Can you work these out from the model? Positions are in its coordinate system, mm. Round coordinates to 2 decimals unless told otherwise and drop trailing zeros. Order: outer loops, then holes, each group sorted by start corner. A loop starts at its lowest first (then second) coordinate and runs counter-clockwise, first axis right, second up. Notation, with made-up numbers: (7, 78.5) -> (38, 78.5) arc R18 ccw to (38, 106.5) -> close; hole circle Ø10 at (62.25, 43). An arc over 180 degrees is marked (long way). Use a Markdown table: item, result. Add a question column.
Q1. If we section it at B-B on y = 19.5: List the corners of the cut face in (x, z) for me.
Q2. I need wall thicknesses on line 1 along Y through (x, z) = (-55, 0.6); line 2 along Y through (x, z) = (33, 0.7) (3 decimals); line 3 along Y through (x, z) = (131.5, 0.3). Which ranges of each line are inside material? Lowest first, please. Write a range as [from, to].
Q3. If we section it at C-C on z = 0.4: Give the number of separate pieces and of enclosed holes in the cut face, plus the area to 3 significant figures.
Q4. If we section it at A-A on x = 22: List the corners of the cut face in (y, z) for me.
Q5. We'd pull the mould along Y, two halves only. Please class faces 1 (the face through (132.801, 134.024, 0.986)), 2 (the face through (2, 162, 0)): +Y half, -Y half, draft (parallel to the pull), parting line (faces both ways), or undercut.
```python
from build123d import *

# Parameters (mm, degrees)
SKETCH_1_R      = 2.05
SKETCH_1_R_2    = 4
SKETCH_1_W      = 8.8
SKETCH_1_H      = 2.8
SKETCH_1_W_2    = 2.5
SKETCH_1_H_2    = 8.5
SKETCH_1_W_3    = 8.5
SKETCH_1_H_3    = 2.5
SKETCH_1_W_4    = 241.301375666
SKETCH_1_H_4    = 241.301375666
SKETCH_1_H_5    = 67.3
EXTRUDE_1_DEPTH = 2


with BuildPart() as part:
    # 草图1 → 凸台-拉伸1 (new body)
    with BuildSketch(Plane.XY):
        Polygon((150.650687833, -150.650687833), (-150.650687833, -150.650687833), (-150.650687833, 150.650687833), (-150.650687833, 277.950687833), (150.650687833, 277.950687833), (150.650687833, 150.650687833), align=None)
        with Locations((0.724285714, -142.895)):
            Circle(SKETCH_1_R, mode=Mode.SUBTRACT)
        with Locations((66.724285714, -142.895)):
            Circle(SKETCH_1_R, mode=Mode.SUBTRACT)
        with Locations(Location((-65.275714286, -142.895, 0), (0, 0, 180))):
            Circle(SKETCH_1_R, mode=Mode.SUBTRACT)
        with Locations(Location((-143.125714286, 66.955, 0), (0, 0, 180))):
            Circle(SKETCH_1_R, mode=Mode.SUBTRACT)
        with Locations((-143.125714286, 0.955)):
            Circle(SKETCH_1_R, mode=Mode.SUBTRACT)
        with Locations((-143.125714286, -65.045)):
            Circle(SKETCH_1_R, mode=Mode.SUBTRACT)
        with Locations(Location((66.874285714, 144.955, 0), (0, 0, 180))):
            Circle(SKETCH_1_R, mode=Mode.SUBTRACT)
        with Locations((0.874285714, 144.955)):
            Circle(SKETCH_1_R, mode=Mode.SUBTRACT)
        with Locations((-65.125714286, 144.955)):
            Circle(SKETCH_1_R, mode=Mode.SUBTRACT)
        with Locations(Location((144.874285714, -65.045, 0), (0, 0, 180))):
            Circle(SKETCH_1_R, mode=Mode.SUBTRACT)
        with Locations((144.874285714, 0.955)):
            Circle(SKETCH_1_R, mode=Mode.SUBTRACT)
        with Locations((144.874285714, 66.955)):
            Circle(SKETCH_1_R, mode=Mode.SUBTRACT)
        with Locations((-130.650687833, -130.650687833)):
            Circle(SKETCH_1_R_2, mode=Mode.SUBTRACT)
        with Locations((-130.650687833, 130.650687833)):
            Circle(SKETCH_1_R_2, mode=Mode.SUBTRACT)
        with Locations((130.650687833, 130.650687833)):
            Circle(SKETCH_1_R_2, mode=Mode.SUBTRACT)
        with Locations((130.650687833, -130.650687833)):
            Circle(SKETCH_1_R_2, mode=Mode.SUBTRACT)
        with Locations((99.724285714, -142.895)):
            Rectangle(SKETCH_1_W, SKETCH_1_H, mode=Mode.SUBTRACT)
        with Locations((33.724285714, -142.895)):
            Rectangle(SKETCH_1_W, SKETCH_1_H, mode=Mode.SUBTRACT)
        with Locations((-32.275714286, -142.895)):
            Rectangle(SKETCH_1_W, SKETCH_1_H, mode=Mode.SUBTRACT)
        with Locations((-98.275714286, -142.895)):
            Rectangle(SKETCH_1_W, SKETCH_1_H, mode=Mode.SUBTRACT)
        with Locations((-143.125714286, 99.955)):
            Rectangle(SKETCH_1_W_2, SKETCH_1_H_2, mode=Mode.SUBTRACT)
        with Locations((-143.125714286, 33.955)):
            Rectangle(SKETCH_1_W_2, SKETCH_1_H_2, mode=Mode.SUBTRACT)
        with Locations((-143.125714286, -32.045)):
            Rectangle(SKETCH_1_W_2, SKETCH_1_H_2, mode=Mode.SUBTRACT)
        with Locations((-143.125714286, -98.045)):
            Rectangle(SKETCH_1_W_2, SKETCH_1_H_2, mode=Mode.SUBTRACT)
        with Locations((99.874285714, 144.955)):
            Rectangle(SKETCH_1_W_3, SKETCH_1_H_3, mode=Mode.SUBTRACT)
        with Locations((33.874285714, 144.955)):
            Rectangle(SKETCH_1_W_3, SKETCH_1_H_3, mode=Mode.SUBTRACT)
        with Locations((-32.125714286, 144.955)):
            Rectangle(SKETCH_1_W_3, SKETCH_1_H_3, mode=Mode.SUBTRACT)
        with Locations((-98.125714286, 144.955)):
            Rectangle(SKETCH_1_W_3, SKETCH_1_H_3, mode=Mode.SUBTRACT)
        with Locations((144.874285714, -98.045)):
            Rectangle(SKETCH_1_W_2, SKETCH_1_H_2, mode=Mode.SUBTRACT)
        with Locations((144.874285714, -32.045)):
            Rectangle(SKETCH_1_W_2, SKETCH_1_H_2, mode=Mode.SUBTRACT)
        with Locations((144.874285714, 33.955)):
            Rectangle(SKETCH_1_W_2, SKETCH_1_H_2, mode=Mode.SUBTRACT)
        with Locations((144.874285714, 99.955)):
            Rectangle(SKETCH_1_W_2, SKETCH_1_H_2, mode=Mode.SUBTRACT)
        Rectangle(SKETCH_1_W_4, SKETCH_1_H_4, mode=Mode.SUBTRACT)
        with Locations((0, 214.300687833)):
            Rectangle(SKETCH_1_W_4, SKETCH_1_H_5, mode=Mode.SUBTRACT)
    extrude(amount=EXTRUDE_1_DEPTH)


solid = part.part
```
Answer below:
| question | item | result |
|---|---|---|
| 1 | outline | (-150.65, 0) -> (-120.65, 0) -> (-120.65, 2) -> (-150.65, 2) -> close; (120.65, 0) -> (150.65, 0) -> (150.65, 2) -> (120.65, 2) -> close |
| 2 | line 1 | [-150.65, -120.65], [120.65, 180.65], [247.95, 277.95] |
| 2 | line 2 | [-150.651, -144.295], [-141.495, -120.651], [120.651, 143.705], [146.205, 180.651], [247.951, 277.951] |
| 2 | line 3 | [-150.65, -134.56], [-126.74, 126.74], [134.56, 277.95] |
| 3 | separate pieces | 1 |
| 3 | enclosed holes | 34 |
| 3 | area | 54,000 mm² |
| 4 | outline | (-150.65, 0) -> (-120.65, 0) -> (-120.65, 2) -> (-150.65, 2) -> close; (120.65, 0) -> (180.65, 0) -> (180.65, 2) -> (120.65, 2) -> close; (247.95, 0) -> (277.95, 0) -> (277.95, 2) -> (247.95, 2) -> close |
| 5 | face 1 | undercut |
| 5 | face 2 | draft |
